Build history of the part. All positions in model axes, mm. Coordinates: 2 decimals unless noted, no trailing zeros.
Item 1: Cut at A-A (z = 3.6). Count the separate pieces of the cut face and the enclosed holes in it, and give its area (3 significant figures).
Item 2: Drill centre lines: line 1 along X through (y, z) = (-51, 1.95); line 2 along X through (y, z) = (-23, 0.5); line 3 along Y through (x, z) = (-75, 0.4). Where is each one in solid material? Low to high.
Item 3: Flat gauge pins, fed straight in: pin 1 (4.5 mm diameter, centred on x = 123.98, y = -116.14, fed in from +Z); pin 2 (2.5 mm diameter, centred on x = -161.5, z = 3, fed in from +Y). Where does each tip first touch, or does it go through?
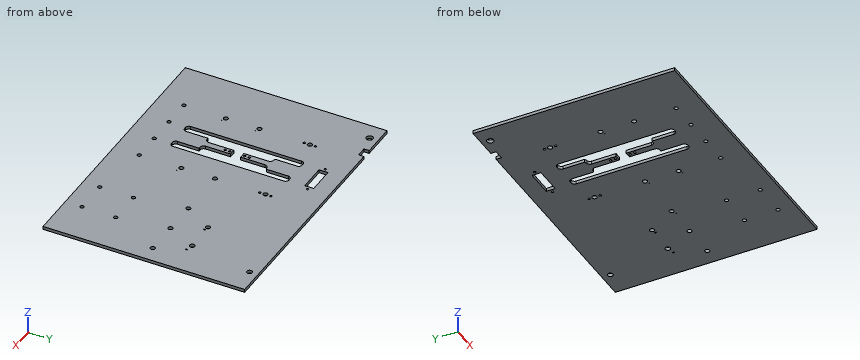
from build123d import *

# Parameters (mm, degrees)
F0_W     = 406.4
F0_H     = 304.8
F1_DEPTH = 4.7625
F2_R     = 1.7399
F2_R_2   = 3.429
F2_R_3   = 3.556
F2_W     = 15.24
F2_H     = 7.874
F2_R_4   = 4.953
F2_R_5   = 3.81
F2_R_6   = 3.937
F2_W_2   = 40.64
F2_H_2   = 13.462
F2_R_7   = 1.651
F3_DEPTH = 25.4
F4_R     = 2.921
F5_DEPTH = 25.4


with BuildPart() as f1:
    # F0 (on Top) → F1 (new body)
    with BuildSketch(Plane.XY):
        with Locations((-15.715082, 10.855626)):
            Rectangle(F0_W, F0_H)
    extrude(amount=F1_DEPTH)

    # F2 (on Top) → F3 (cut)
    with BuildSketch(Plane.XY):
        with Locations((-142.715082, 95.437626)):
            Circle(F2_R)
        with Locations((-142.715082, 78.673626)):
            Circle(F2_R)
        with Locations((-142.715082, 10.855626)):
            Circle(F2_R_2)
        with Locations((-142.715082, 87.055626)):
            Circle(F2_R_3)
        Polygon((-135.356732, 7.724144), (-136.59422, 8.009667), (-136.672544, 7.670205), (-135.435056, 7.384682), align=None)
        with Locations((-142.715082, -39.944374)):
            Circle(F2_R_2)
        Polygon((-135.356732, -43.075856), (-136.59422, -42.790333), (-136.672544, -43.129795), (-135.435056, -43.415318), align=None)
        with Locations((-15.715082, -39.944374)):
            Circle(F2_R_2)
        with Locations((-15.715082, 87.055626)):
            Circle(F2_R_3)
        with Locations((-15.715082, 10.855626)):
            Circle(F2_R_2)
        with Locations((-15.715082, 78.673626)):
            Circle(F2_R)
        with Locations((-15.715082, 95.437626)):
            Circle(F2_R)
        Polygon((-8.435056, 7.384682), (-8.356732, 7.724144), (-9.59422, 8.009667), (-9.672544, 7.670205), align=None)
        Polygon((-8.435056, -43.415318), (-8.356732, -43.075856), (-9.59422, -42.790333), (-9.672544, -43.129795), align=None)
        with Locations((-160.495082, 159.318626)):
            Rectangle(F2_W, F2_H)
        with Locations((-193.515082, 150.555626)):
            Circle(F2_R_4)
        Polygon((67.764944, 7.384682), (67.843268, 7.724144), (66.60578, 8.009667), (66.527456, 7.670205), align=None)
        with Locations((60.484918, 10.855626)):
            Circle(F2_R_2)
        Polygon((117.40578, 8.009667), (117.327456, 7.670205), (118.564944, 7.384682), (118.643268, 7.724144), align=None)
        with Locations((111.284918, 10.855626)):
            Circle(F2_R_2)
        Polygon((168.20578, 8.009667), (168.127456, 7.670205), (169.364944, 7.384682), (169.443268, 7.724144), align=None)
        with Locations((162.084918, 10.855626)):
            Circle(F2_R_2)
        Polygon((94.038508, 53.655909), (92.80102, 53.941433), (92.172868, 51.218959), (93.410356, 50.933436), align=None)
        with Locations((86.052007, 54.064918)):
            Circle(F2_R_2)
        Polygon((144.838508, 53.655909), (143.60102, 53.941433), (142.972868, 51.218959), (144.210356, 50.933436), align=None)
        with Locations((132.892046, 54.978594)):
            Circle(F2_R_5)
        with BuildLine():
            Line((-96.995082, 99.755626), (-99.535082, 99.755626))
            ThreePointArc((-99.535082, 99.755626), (-103.127184, 98.267729), (-104.615082, 94.675626))
            Line((-104.615082, 94.675626), (-104.615082, -72.964374))
            ThreePointArc((-104.615082, -72.964374), (-103.127184, -76.556476), (-99.535082, -78.044374))
            Line((-99.535082, -78.044374), (-96.995082, -78.044374))
            ThreePointArc((-96.995082, -78.044374), (-93.402979, -76.556476), (-91.915082, -72.964374))
            Line((-91.915082, -72.964374), (-91.915082, -39.944374))
            Line((-91.915082, -39.944374), (-89.606103, -39.944374))
            Line((-89.606103, -39.944374), (-88.955982, -39.944374))
            ThreePointArc((-88.955982, -39.944374), (-85.363879, -38.456476), (-83.875982, -34.864374))
            Line((-83.875982, -34.864374), (-83.875982, 1.199732))
            Line((-83.875982, 1.199732), (-83.875982, 3.235626))
            Line((-83.875982, 3.235626), (-74.554182, 3.235626))
            Line((-74.554182, 3.235626), (-74.554182, -34.864374))
            ThreePointArc((-74.554182, -34.864374), (-73.066284, -38.456476), (-69.474182, -39.944374))
            Line((-69.474182, -39.944374), (-68.82406, -39.944374))
            Line((-68.82406, -39.944374), (-66.515082, -39.944374))
            Line((-66.515082, -39.944374), (-66.515082, -72.964374))
            ThreePointArc((-66.515082, -72.964374), (-65.027184, -76.556476), (-61.435082, -78.044374))
            Line((-61.435082, -78.044374), (-58.895082, -78.044374))
            ThreePointArc((-58.895082, -78.044374), (-55.302979, -76.556476), (-53.815082, -72.964374))
            Line((-53.815082, -72.964374), (-53.815082, 94.675626))
            ThreePointArc((-53.815082, 94.675626), (-55.302979, 98.267729), (-58.895082, 99.755626))
            Line((-58.895082, 99.755626), (-61.435082, 99.755626))
            ThreePointArc((-61.435082, 99.755626), (-65.027184, 98.267729), (-66.515082, 94.675626))
            Line((-66.515082, 94.675626), (-66.515082, 61.655626))
            Line((-66.515082, 61.655626), (-71.004661, 60.237118))
            ThreePointArc((-71.004661, 60.237118), (-73.571817, 58.395778), (-74.554182, 55.393149))
            Line((-74.554182, 55.393149), (-74.554182, 18.475626))
            Line((-74.554182, 18.475626), (-83.875982, 18.475626))
            Line((-83.875982, 18.475626), (-83.875982, 55.393149))
            ThreePointArc((-83.875982, 55.393149), (-84.858346, 58.395778), (-87.425502, 60.237118))
            Line((-87.425502, 60.237118), (-91.915082, 61.655626))
            Line((-91.915082, 61.655626), (-91.915082, 94.675626))
            ThreePointArc((-91.915082, 94.675626), (-93.402979, 98.267729), (-96.995082, 99.755626))
        make_face()
        with Locations((-79.215082, 21.930026)):
            Circle(F2_R)
        with Locations((-79.215082, 29.245226)):
            Circle(F2_R)
        with Locations((-79.215082, -7.533974)):
            Circle(F2_R)
        with Locations((-79.215082, -0.218774)):
            Circle(F2_R)
        with Locations((149.384918, 150.555626)):
            Circle(F2_R_6)
        with Locations((-77.945082, 131.124626)):
            Rectangle(F2_W_2, F2_H_2)
        with Locations((-52.545082, 131.124626)):
            Circle(F2_R_7)
        with Locations((-103.345082, 131.124626)):
            Circle(F2_R_7)
    extrude(amount=F3_DEPTH, mode=Mode.SUBTRACT)

    # F4 (on face) → F5 (cut)
    with BuildSketch(Plane.XY.offset(4.7625)):
        with Locations((-142.715082, -103.444374)):
            Circle(F4_R)
        with Locations((-100.297082, -103.444374)):
            Circle(F4_R)
        with Locations((73.184918, -65.344374)):
            Circle(F4_R)
        with Locations((73.184918, -116.144374)):
            Circle(F4_R)
        with Locations((123.984918, -65.344374)):
            Circle(F4_R)
        with Locations((123.984918, -116.144374)):
            Circle(F4_R)
        with Locations((-57.879082, -103.444374)):
            Circle(F4_R)
        with Locations((-15.461082, -103.444374)):
            Circle(F4_R)
    extrude(amount=-F5_DEPTH, mode=Mode.SUBTRACT)


solid = f1.part
Filled sheet:
1. separate pieces: 1
1. enclosed holes: 42
1. area: 116,000 mm2
2. line 1: x = -218.92 to -104.62, -91.92 to -66.52, -53.82 to 187.48
2. line 2: x = -218.92 to -104.62, -83.88 to -74.55, -53.82 to 187.48
2. line 3: y = -141.54 to 3.24, 18.48 to 124.39, 137.86 to 163.26
3. pin 1: passes through
3. pin 2: stops at y = 155.38
